```python
from build123d import *

# Parameters (mm, degrees)
EXTRUDE_THIN1_DEPTH = 349.25
FILLET1_R           = 1.27


with BuildPart() as part:
    # Sketch1 → Extrude-Thin1 (new body)
    with BuildSketch(Plane.XY):
        with BuildLine():
            Line((0, 34.925), (-17.4625, 34.925))
            Line((-17.4625, 34.925), (-17.4625, 19.05))
            Line((-17.4625, 19.05), (-12.7, 19.05))
            ThreePointArc((-12.7, 19.05), (-11.5566064, 13.811099671), (-8.334375, 9.525))
            ThreePointArc((-8.334375, 9.525), (-5.1121436, 5.238900329), (-3.96875, 0))
            Line((-3.96875, 0), (0, 0))
            Line((0, 0), (0, 1.27))
            Line((0, 1.27), (-2.757126928, 1.27))
            ThreePointArc((-2.757126928, 1.27), (-4.23576048, 6.339833525), (-7.505321915, 10.487065997))
            ThreePointArc((-7.505321915, 10.487065997), (-10.650811196, 14.925884165), (-11.358429664, 20.32))
            Line((-11.358429664, 20.32), (-16.1925, 20.32))
            Line((-16.1925, 20.32), (-16.1925, 33.655))
            Line((-16.1925, 33.655), (0, 33.655))
            Line((0, 33.655), (0, 34.925))
        make_face()
    extrude(amount=-EXTRUDE_THIN1_DEPTH)

    # Fillet1
    fillet1_edges = [part.edges().sort_by_distance(p)[0] for p in [
        (-3.96875, 0, -174.625),
        (-17.4625, 19.05, -174.625),
        (-17.4625, 34.925, -174.625),
        (-11.358429664, 20.32, -174.625),
    ]]
    fillet(fillet1_edges, radius=FILLET1_R)


solid = part.part
```
Verification items for the finished model (mm, model axes). A direction names the side the tool comes from. Coordinates: 2 decimals unless noted, no trailing zeros. Order: outer loops, then holes, each group sorted by start corner. A loop starts at its lowest first (then second) coordinate and runs counter-clockwise, first axis right, second up. Notation, with made-up numbers: (3.5, -39.75) - (13.5, -39.75) arc R28 cw to (13.5, -7.75) - close; hole circle Ø8 at (50.25, 47). An arc over 180 degrees is marked (long way). Return JSON: item names as keys, results as strings.
(1) Mould release check, pull along Y, two halves, no side actions. Record for faces 3 (the flat face through (-16.192, 27, -172)), 4 (the flat face through (-8, 33.655, -172)), 5 (the flat face through (-8, 34.925, -172)), 6 (the flat face through (-17.462, 27, -172)): pulls with the +Y half, pulls with the -Y half, needs draft (parallel to the pull), parting line crosses it, or undercut.
Filled sheet:
{"face 3": "undercut", "face 4": "undercut", "face 5": "pulls with the +Y half", "face 6": "needs draft"}
(2) Thickness scan on line 1 along Y through (x, z) = (-1.5, -245) (3 decimals); line 2 along X through (y, z) = (28, -261); line 3 along X through (y, z) = (19, -299.5). Record the ranges inside material, lowest first.
Filled sheet:
{"line 1": "y = 0 to 1.27, 33.655 to 34.925", "line 2": "x = -17.46 to -16.19", "line 3": "x = -12.7 to -11.43"}
(3) Go/stop test with flat-tipped pins: pin 1 (1 mm diameter, centred on x = -15, z = -249.5, fed in from -Y); pin 2 (5 mm diameter, centred on y = 18, z = -260, fed in from +X); pin 3 (6.5 mm diameter, centred on y = 28.5, z = -109, fed in from +X). Record where each tip stops, or that it passes through.
Filled sheet:
{"pin 1": "stops at y = 19.05", "pin 2": "stops at x = -10.86", "pin 3": "stops at x = -16.19"}
(4) Access from +Z, -Z, +X, -X, +Y, -Y to the whole of each face (thin tool, end or side, straight path). Record for faces 1 (the cylindrical face through (-10.374, 14.279, -172.18)), 2 (the flat face through (-13, 20, -349.25)).
Filled sheet:
{"face 1": "+Z, -Z, +X", "face 2": "-Z, +X, -X, +Y, -Y"}
(5) Section check B-B, the plane y = 26. Record the cut outline in (x, z), and give its area (3 significant figures).
Filled sheet:
{"outline": "(-17.46, -349.25) - (-16.19, -349.25) - (-16.19, 0) - (-17.46, 0) - close", "area": "444 mm^2"}
